Geometry: final body of the model. Coordinates: model frame, mm. A direction names the side the tool comes from. Give positions to 0.01 mm unless a question says otherwise; leave off trailing zeros. Loops run counter-clockwise (first coordinate to the right, second up) from the corner with the lowest first, then second, coordinate; pieces in that order, holes last. Notation, with made-up numbers: (22.25, 20.25) -> (52.25, 20.25) arc R21 ccw to (52.25, 50.25) -> close; hole circle Ø5 at (72, 38.5). An arc over 180 degrees is marked (long way). Answer in a Markdown table with one row per item. Add a question column.
from build123d import *

# Parameters (mm, degrees)
SKETCH1_R           = 68.659375
SKETCH1_R_2         = 55.959375
BOSS_EXTRUDE1_DEPTH = 3.175
BOSS_EXTRUDE2_START = -3.175
BOSS_EXTRUDE2_DEPTH = 3.175
CIRPATTERN1_COUNT   = 9
SKETCH3_R           = 2.2225
BOSS_EXTRUDE3_DEPTH = 6.35
CIRPATTERN13_COUNT  = 9


with BuildPart() as part:
    # Sketch1 → Boss-Extrude1 (new body)
    with BuildSketch(Plane(origin=(0, 0, 0), x_dir=(1, 0, 0), z_dir=(0, 1, 0))):
        with Locations(Location((0, 0, 0), (0, 0, 270))):
            Circle(SKETCH1_R)
        with Locations(Location((0, 0, 0), (0, 0, 270))):
            Circle(SKETCH1_R_2, mode=Mode.SUBTRACT)
    extrude(amount=BOSS_EXTRUDE1_DEPTH)

    # Sketch2 → Boss-Extrude2 (add)
    with BuildSketch(Plane(origin=(0, 3.175, 0), x_dir=(1, 0, 0), z_dir=(0, 1, 0)).offset(BOSS_EXTRUDE2_START)):
        with BuildLine():
            Line((-4.653697789, 71.001707707), (-5.372788209, 81.972907412))
            ThreePointArc((-5.372788209, 81.972907412), (0, 87.709375), (5.372788209, 81.972907412))
            ThreePointArc((5.372788209, 81.972907412), (1.580107525, 80.725221164), (0.983574692, 76.777399446))
            Line((0.983574692, 76.777399446), (3.889375, 69.933810414))
            ThreePointArc((3.889375, 69.933810414), (4.734169071, 68.871766239), (6.005193091, 68.39625305))
            ThreePointArc((6.005193091, 68.39625305), (-0.46538454, 68.657797755), (-6.931822104, 68.308561818))
            ThreePointArc((-6.931822104, 68.308561818), (-5.249012804, 69.195180628), (-4.653697789, 71.001707707))
        make_face()
    boss_extrude2 = extrude(amount=BOSS_EXTRUDE2_DEPTH)

    # CirPattern1: Boss-Extrude2 ×9 about axis
    cirpattern1_axis = Axis((0, 0, 0), (0, 1, 0))
    for i in range(1, CIRPATTERN1_COUNT):
        add(boss_extrude2.rotate(cirpattern1_axis, i * 360 / CIRPATTERN1_COUNT))

    # Sketch3 → Boss-Extrude3 (add)
    with BuildSketch(Plane(origin=(0, 3.175, 0), x_dir=(1, 0, 0), z_dir=(0, 1, 0))):
        with Locations(Location((0, 84.132166, 0), (0, 0, 270))):
            Circle(SKETCH3_R)
    boss_extrude3 = extrude(amount=-BOSS_EXTRUDE3_DEPTH)

    # CirPattern13: Boss-Extrude3 ×9 about axis
    cirpattern13_axis = Axis((0, 0, 0), (0, 1, 0))
    for i in range(1, CIRPATTERN13_COUNT):
        add(boss_extrude3.rotate(cirpattern13_axis, i * 360 / CIRPATTERN13_COUNT))


solid = part.part
(1) Cut plane A-A on z = 0. Return the cut outline in (x, y) (3 decimals).
(2) Cut plane B-B on x = -37. Return the cut outline in (y, z) (3 decimals).
(3) Pin query (flat end, axial travel): pin 1 Ø1.5 at (x, y) = (-53, -0.5) entering from -Z; pin 2 Ø4 at (x, z) = (51.5, 26) entering from -Y; pin 3 Ø3 at (y, z) = (1.5, 29) entering from +X. Return the tip coordinate at first contact, or that it passes through.
(4) Material intervals for line 1 along X through (y, z) = (1.25, 41); line 2 along X through (y, z) = (3, -1.5); line 3 along X through (y, z) = (1.85, 0), sorted ascending. Write a range as from..to.
(5) Reachability of faces 4 (the flat face through (73, -3.175, 42)), 5 (the flat face through (72.71, 1.57, -10.37)), 6 (the cylindrical face through (-85.024, -1.565, -15.091)), 7 (the flat face through (45.279, 1.565, -61.753)) from +Z, -Z, +X, -X, +Y, -Y: full face, straight path, thin tool, end or side. Return the list, or none.
(6) Draft query along Z for faces 1 (the flat face through (-73, -3.175, 42)), 2 (the cylindrical face through (-29.146, 1.565, 75.345)), 3 (the cylindrical face through (72.958, -1.565, 39.846)). Return one class per face: +Z half, -Z half, draft (parallel to the pull), parting line (faces both ways), or undercut.
(7) Cut plane C-C on z = -73.5. Return the cut outline in (x, y) (3 decimals), then the cut area to 3 significant figures.
Answer list:
| question | item | result |
|---|---|---|
| 1 | outline | (-68.659, 0) -> (-55.959, 0) -> (-55.959, 3.175) -> (-68.659, 3.175) -> close; (55.959, 0) -> (68.659, 0) -> (68.659, 3.175) -> (55.959, 3.175) -> close |
| 2 | outline | (0, -57.837) -> (3.175, -57.837) -> (3.175, -41.982) -> (0, -41.982) -> close; (0, 41.982) -> (3.175, 41.982) -> (3.175, 57.837) -> (0, 57.837) -> close |
| 3 | pin 1 | stops at z = -68.45 |
| 3 | pin 2 | stops at y = 0 |
| 3 | pin 3 | stops at x = 62.91 |
| 4 | line 1 | x = -76.68..-61.36, -55.07..-38.08, 38.08..55.07, 68.76..76.68 |
| 4 | line 2 | x = -68.64..-55.94, 55.94..68.64 |
| 4 | line 3 | x = -68.66..-55.96, 55.96..68.66 |
| 5 | face 4 | +Z, -Z, +X, -X, -Y |
| 5 | face 5 | +Y, -Y |
| 5 | face 6 | -Y |
| 5 | face 7 | -Z, +Y, -Y |
| 6 | face 1 | draft |
| 6 | face 2 | undercut |
| 6 | face 3 | parting line |
| 7 | outline | (-4.817, 0) -> (2.375, 0) -> (2.375, 3.175) -> (-4.817, 3.175) -> close |
| 7 | area | 22.8 mm² |
